```python
from build123d import *

# Parameters (mm, degrees)
SKETCH1_R          = 12.5
SKETCH1_R_2        = 1.6
EXTRUDE1_DEPTH     = 3
CHAMFER1_SIZE      = 20
SKETCH2_R          = 1.6
CUT_EXTRUDE1_DEPTH = 3
CUT_EXTRUDE3_DEPTH = 3


with BuildPart() as part:
    # Sketch1 → Extrude1 (new body)
    with BuildSketch(Plane.XY):
        with BuildLine():
            Line((77.718550226, 11.3466222), (53.857627652, 58.447539112))
            Line((53.857627652, 58.447539112), (9.254486637, 35.851968493))
            Line((9.254486637, 35.851968493), (-13.637193397, 20.952970106))
            ThreePointArc((-13.637193397, 20.952970106), (-21.658878744, -12.485710694), (11.29778531, -22.301570507))
            Line((11.29778531, -22.301570507), (77.718550226, 11.3466222))
        make_face()
        Circle(SKETCH1_R, mode=Mode.SUBTRACT)
        with Locations((53.476276267, 45.923379615)):
            Circle(SKETCH1_R_2, mode=Mode.SUBTRACT)
        with Locations((42.771522423, 40.500442666)):
            Circle(SKETCH1_R_2, mode=Mode.SUBTRACT)
        with BuildLine():
            Line((8.126668077, 16.37149411), (7.222845253, 18.15561975))
            ThreePointArc((7.222845253, 18.15561975), (8.147163209, 20.977965639), (10.969509098, 20.053647682))
            Line((10.969509098, 20.053647682), (11.873331923, 18.269522042))
            ThreePointArc((11.873331923, 18.269522042), (10.949013966, 15.447176153), (8.126668077, 16.37149411))
        make_face(mode=Mode.SUBTRACT)
        with BuildLine():
            Line((-21.873331923, -0.949013966), (-22.777154747, 0.835111675))
            ThreePointArc((-22.777154747, 0.835111675), (-21.852836791, 3.657457563), (-19.030490902, 2.733139607))
            Line((-19.030490902, 2.733139607), (-18.126668077, 0.949013966))
            ThreePointArc((-18.126668077, 0.949013966), (-19.050986034, -1.873331923), (-21.873331923, -0.949013966))
        make_face(mode=Mode.SUBTRACT)
        with BuildLine():
            Line((8.126668077, -18.269522042), (7.222845253, -16.485396401))
            ThreePointArc((7.222845253, -16.485396401), (8.147163209, -13.663050512), (10.969509098, -14.587368469))
            Line((10.969509098, -14.587368469), (11.873331923, -16.37149411))
            ThreePointArc((11.873331923, -16.37149411), (10.949013966, -19.193839998), (8.126668077, -18.269522042))
        make_face(mode=Mode.SUBTRACT)
    extrude(amount=EXTRUDE1_DEPTH)

    # Chamfer1
    chamfer1_edges = [part.edges().sort_by_distance(p)[0] for p in [
        (77.718550226, 11.3466222, 1.5),
    ]]
    chamfer(chamfer1_edges, length=CHAMFER1_SIZE)

    # Sketch2 → Cut-Extrude1 (cut)
    with BuildSketch(Plane.XY.offset(3)):
        with Locations((62.526264519, 25.846086156)):
            Circle(SKETCH2_R)
        with Locations((49.145322214, 19.06741497)):
            Circle(SKETCH2_R)
        with Locations((43.188041489, 1.899305514)):
            Circle(SKETCH2_R)
    extrude(amount=-CUT_EXTRUDE1_DEPTH, mode=Mode.SUBTRACT)

    # Sketch4 → Cut-Extrude3 (cut)
    with BuildSketch(Plane.XY.offset(3)):
        with BuildLine():
            Line((20.102322982, 24.532430534), (47.488856964, 38.406214947))
            ThreePointArc((47.488856964, 38.406214947), (48.918221015, 38.11442299), (48.960317371, 36.656187058))
            Line((48.960317371, 36.656187058), (21.573783389, -0.017867108))
            ThreePointArc((21.573783389, -0.017867108), (20.262801724, -0.42963276), (19.458756207, 0.684698738))
            Line((19.458756207, 0.684698738), (19.458756207, 23.48496849))
            ThreePointArc((19.458756207, 23.48496849), (19.63250249, 24.099654371), (20.102322982, 24.532430534))
        make_face()
    extrude(amount=-CUT_EXTRUDE3_DEPTH, mode=Mode.SUBTRACT)


solid = part.part
```
Design review of the part built by this model. Coordinates are the model's own, in mm. A direction names the side the tool comes from. Give positions to 0.01 mm unless a question says otherwise; leave off trailing zeros. Order: outer loops, then holes, each group sorted by start corner. A loop starts at its lowest first (then second) coordinate and runs counter-clockwise, first axis right, second up. Notation, with made-up numbers: (-19.5, 36.5) - (3.5, 36.5) arc R19 ccw to (3.5, 52.5) - close; hole circle Ø5 at (3.25, 81). An arc over 180 degrees is marked (long way). Use a Markdown table: item, result. Add a question column.
(1) Add section B-B on y = 33.5. Give the boundary of the cut face in (x, z).
(2) Add section A-A on x = 3. Give the boundary of the cut face in (y, z).
(3) Mouldability with a two-part tool opening along X and no side actions: class faces 3 (the face through (-2.031, 28.507, 1.479)), 4 (the face through (32, 8, 0)), 5 (the face through (8.106, -13.684, 1.479)) as +X half, -X half, draft (parallel to the pull), parting line (faces both ways), or undercut.
(4) Machinability: for faces 1 (the face through (64.217, 15.56, 1.479)), 2 (the face through (19.459, 12, 2)), which of the approach directions +Z, -Z, +X, -X, +Y, -Y give a long, thin tool a straight path to every point of the face, cutting with its end or side? Answer none if there is none.
(5) Add section C-C on z = 2.35. Give the number of separate pieces and of enclosed holes in the cut face, then the cut area to 3 significant figures.
(6) Wall thickness on probe 1 along X at (y, z) = (4, 1.3); probe 2 along X at (y, z) = (26, 1.45); probe 3 along Y at (x, z) = (42.5, 1.2) (3 decimals): over which ranges is each line inside the solid? List them lowest first. Write a range as [from, to].
Report:
| question | item | result |
|---|---|---|
| 1 | outline | (5.64, 0) - (37.8, 0) - (37.8, 3) - (5.64, 3) - close; (46.6, 0) - (66.5, 0) - (66.5, 3) - (46.6, 3) - close |
| 2 | outline | (-24.82, 0) - (-12.13, 0) - (-12.13, 3) - (-24.82, 3) - close; (12.13, 0) - (31.78, 0) - (31.78, 3) - (12.13, 3) - close |
| 3 | face 3 | -X half |
| 3 | face 4 | draft |
| 3 | face 5 | undercut |
| 4 | face 1 | +Z, -Z, +X, -Y |
| 4 | face 2 | +Z, -Z |
| 5 | separate pieces | 1 |
| 5 | enclosed holes | 10 |
| 5 | area | 3,650 mm² |
| 6 | probe 1 | x = [-24.68, -11.84], [11.84, 19.46], [24.57, 60.43] |
| 6 | probe 2 | x = [-5.88, 23], [41, 60.93], [64.12, 67.64] |
| 6 | probe 3 | y = [-6.495, 0.455], [3.344, 28.005], [35.879, 38.924], [42.077, 52.694] |
